Part print with two shaded views. Sizes in mm from the minimum x, y, z corner. A direction names the side the tool comes from. Round coordinates to 2 decimals unless told otherwise and drop trailing zeros. Loops run counter-clockwise (first coordinate to the right, second up) from the corner with the lowest first, then second, coordinate; pieces in that order, holes last. Notation, with made-up numbers: (26, 58.25) - (34, 58.25) arc R12 cw to (34, 81.25) - close; hole circle Ø7 at (-8.75, 59.5). An arc over 180 degrees is marked (long way). One line per question, with ' | ' between items.
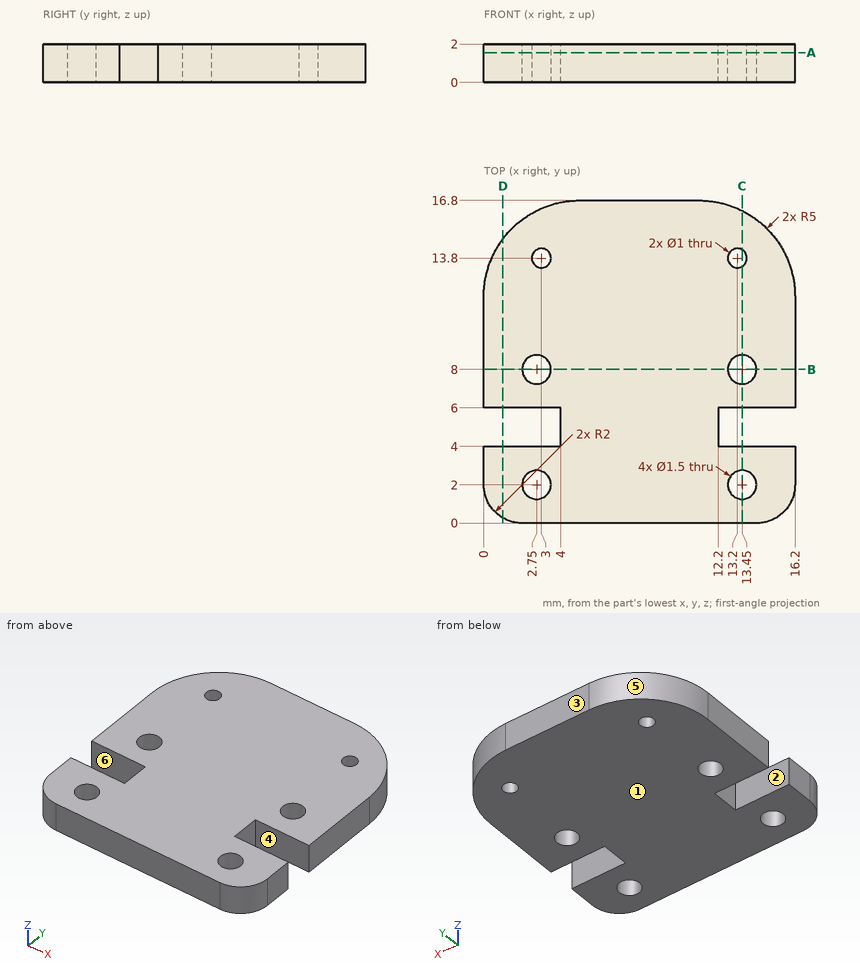
(1) Drop flat-ended pins along their axis: P1, Ø0.6, axis at x = 2, z = 1.5, coming from the +Y side; P2, Ø0.6, axis at x = 1, z = 1, coming from the -Y side. Give the stop position or say it passes through.
Results found:
P1: stops at y = 16.01 | P2: stops at y = 0.13
(2) Cut at B-B, the plane y = 8. Write the cut outline in (x, z), then the cut area to 3 significant figures.
Results found:
outline: (0, 0) - (2, 0) - (2, 2) - (0, 2) - close; (3.5, 0) - (12.7, 0) - (12.7, 2) - (3.5, 2) - close; (14.2, 0) - (16.2, 0) - (16.2, 2) - (14.2, 2) - close | area: 26.4 mm²
(3) Two-plate mould, pull along Y, no slides. Class the marked faces 1, 2 and 3: released by +Y, released by -Y, zero draft, split by the parting line, or undercut.
Results found:
face 1: zero draft | face 2: undercut | face 3: released by +Y
(4) Tool access for the marked faces 4, 5 and 6: list every direction of +Z, -Z, +X, -X, +Y, -Y with a clear straight run to the whole face (end or side of a thin tool).
Results found:
face 4: +Z, -Z, +X | face 5: +Z, -Z, -X, +Y | face 6: +Z, -Z, -X
(5) Cut at C-C, the plane x = 13.45. Write the cut outline in (y, z).
Results found:
outline: (0, 0) - (1.25, 0) - (1.25, 2) - (0, 2) - close; (2.75, 0) - (4, 0) - (4, 2) - (2.75, 2) - close; (6, 0) - (7.25, 0) - (7.25, 2) - (6, 2) - close; (8.75, 0) - (13.37, 0) - (13.37, 2) - (8.75, 2) - close; (14.23, 0) - (16.27, 0) - (16.27, 2) - (14.23, 2) - close
(6) Cut at A-A, the plane z = 1.55. Write the cut outline in (x, y), then the cut area to 3 significant figures.
Results found:
outline: (0, 2) arc R2 ccw to (2, 0) - (14.2, 0) arc R2 ccw to (16.2, 2) - (16.2, 4) - (12.2, 4) - (12.2, 6) - (16.2, 6) - (16.2, 11.8) arc R5 ccw to (11.2, 16.8) - (5, 16.8) arc R5 ccw to (0, 11.8) - (0, 6) - (4, 6) - (4, 4) - (0, 4) - close; hole circle Ø1.5 at (2.75, 2); hole circle Ø1.5 at (2.75, 8); hole circle Ø1 at (3, 13.8); hole circle Ø1.5 at (13.45, 2); hole circle Ø1.5 at (13.45, 8); hole circle Ø1 at (13.2, 13.8) | area: 235 mm²
(7) Cut at D-D, the plane x = 1. Write the cut outline in (y, z), then the cut area to 3 significant figures.
Results found:
outline: (0.27, 0) - (4, 0) - (4, 2) - (0.27, 2) - close; (6, 0) - (14.8, 0) - (14.8, 2) - (6, 2) - close | area: 25.1 mm²
(8) Probe L1, parallel to X at y = 8, z = 0.55; L2, parallel to X at y = 14, z = 1.5; L3, parallel to Y at x = 2.75, z = 0.95. List the from-to ranges inside material, lowest first.
Results found:
L1: x = 0 to 2, 3.5 to 12.7, 14.2 to 16.2 | L2: x = 0.51 to 2.54, 3.46 to 12.74, 13.66 to 15.69 | L3: y = 0 to 1.25, 2.75 to 4, 6 to 7.25, 8.75 to 13.37, 14.23 to 16.27
